```python
from build123d import *

# Parameters (mm, degrees)
SKETCH1_R           = 1.524
SKETCH1_R_2         = 2.4892
SKETCH1_R_3         = 11.522750336
SKETCH1_R_4         = 3.302
BOSS_EXTRUDE1_DEPTH = 6.35
CHAMFER1_SIZE       = 1.905
SKETCH2_R           = 1.1303
CUT_EXTRUDE1_DEPTH  = 12.7


with BuildPart() as part:
    # Sketch1 → Boss-Extrude1 (new body)
    with BuildSketch(Plane(origin=(0, 0, 0), x_dir=(1, 0, 0), z_dir=(0, 1, 0))):
        with BuildLine():
            Line((-48.989983611, 25.571283439), (-67.720507172, 29.04547214))
            Line((-67.720507172, 29.04547214), (-68.878570072, 22.801964286))
            Line((-68.878570072, 22.801964286), (-87.609093633, 26.276152988))
            Line((-87.609093633, 26.276152988), (-86.451030733, 32.519660841))
            Line((-86.451030733, 32.519660841), (-105.181554294, 35.993849543))
            Line((-105.181554294, 35.993849543), (-123.386535507, 39.370559213))
            Line((-123.386535507, 39.370559213), (-143.61245558, 43.122118146))
            Line((-143.61245558, 43.122118146), (-173.397808446, 32.126880331))
            Line((-173.397808446, 32.126880331), (-164.230158466, -34.209448348))
            Line((-164.230158466, -34.209448348), (-143.692879271, -77.813892282))
            Line((-143.692879271, -77.813892282), (-76.563330949, -77.813892282))
            Line((-76.563330949, -77.813892282), (-49.204879271, -77.813892282))
            Line((-49.204879271, -77.813892282), (-49.204879271, -37.681892282))
            Line((-49.204879271, -37.681892282), (45.277962712, -37.681892282))
            Line((45.277962712, -37.681892282), (64.72671994, -37.681892282))
            ThreePointArc((64.72671994, -37.681892282), (47.456106683, -24.721818432), (40.256527969, -4.364911427))
            ThreePointArc((40.256527969, -4.364911427), (40.224315343, -2.464216219), (40.304028245, -0.564920092))
            ThreePointArc((40.304028245, -0.564920092), (40.358687129, 0.79375425), (40.328560009, 2.153193811))
            ThreePointArc((40.328560009, 2.153193811), (38.274981353, 12.886225143), (33.41911498, 22.675796566))
            ThreePointArc((33.41911498, 22.675796566), (30.929713329, 27.951337515), (30.171477502, 33.73524029))
            ThreePointArc((30.171477502, 33.73524029), (27.651370411, 37.853265988), (22.862043617, 37.243820127))
            ThreePointArc((22.862043617, 37.243820127), (20.166682607, 36.055874133), (17.256896531, 36.513401897))
            ThreePointArc((17.256896531, 36.513401897), (8.843040964, 39.405959226), (0, 40.386))
            ThreePointArc((0, 40.386), (-9.489488111, 40.375548652), (-18.94466273, 39.569219451))
            ThreePointArc((-18.94466273, 39.569219451), (-22.43398811, 39.812343861), (-25.563809609, 41.373983535))
            ThreePointArc((-25.563809609, 41.373983535), (-32.045487778, 43.349075748), (-38.20024979, 40.514989348))
            ThreePointArc((-38.20024979, 40.514989348), (-40.550934903, 36.930082806), (-41.360215512, 32.720291801))
            ThreePointArc((-41.360215512, 32.720291801), (-43.17208429, 27.008072674), (-48.989983611, 25.571283439))
        make_face()
        with Locations(Location((-131.808500509, 37.703534036, 0), (0, 0, 270))):
            Circle(SKETCH1_R, mode=Mode.SUBTRACT)
        with Locations(Location((-31.399492492, 33.846007028, 0), (0, 0, 270))):
            Circle(SKETCH1_R, mode=Mode.SUBTRACT)
        with Locations(Location((-23.788932991, -8.902059713, 0), (0, 0, 270))):
            Circle(SKETCH1_R_2, mode=Mode.SUBTRACT)
        with Locations(Location((8.902059713, -23.788932991, 0), (0, 0, 270))):
            Circle(SKETCH1_R_2, mode=Mode.SUBTRACT)
        with Locations(Location((-8.902059713, 23.788932991, 0), (0, 0, 270))):
            Circle(SKETCH1_R_2, mode=Mode.SUBTRACT)
        with Locations(Location((23.788932991, 8.902059713, 0), (0, 0, 270))):
            Circle(SKETCH1_R_2, mode=Mode.SUBTRACT)
        with Locations(Location((0, 0, 0), (0, 0, 270))):
            Circle(SKETCH1_R_3, mode=Mode.SUBTRACT)
        with Locations(Location((-74.604879271, -57.747892282, 0), (0, 0, 270))):
            Circle(SKETCH1_R_4, mode=Mode.SUBTRACT)
        with Locations(Location((-40.020695033, -13.367428306, 0), (0, 0, 270))):
            Circle(SKETCH1_R, mode=Mode.SUBTRACT)
        with Locations(Location((25.727857837, 33.846007028, 0), (0, 0, 270))):
            Circle(SKETCH1_R, mode=Mode.SUBTRACT)
        with BuildLine():
            Line((-142.716614997, 32.622661546), (-162.215024972, 25.424839998))
            Line((-162.215024972, 25.424839998), (-156.726187504, -14.291916991))
            ThreePointArc((-156.726187504, -14.291916991), (-128.01028366, 5.891204618), (-94.602827713, 16.657049623))
            ThreePointArc((-94.602827713, 16.657049623), (-91.648290045, 20.089389422), (-94.519859105, 23.59143746))
            Line((-94.519859105, 23.59143746), (-142.716614997, 32.622661546))
        make_face(mode=Mode.SUBTRACT)
        with BuildLine():
            Line((-114.508797405, -72.415483536), (-119.588797405, -72.415483536))
            ThreePointArc((-119.588797405, -72.415483536), (-124.351297405, -67.652983536), (-119.588797405, -62.890483536))
            Line((-119.588797405, -62.890483536), (-114.508797405, -62.890483536))
            ThreePointArc((-114.508797405, -62.890483536), (-109.746297405, -67.652983536), (-114.508797405, -72.415483536))
        make_face(mode=Mode.SUBTRACT)
        with BuildLine():
            ThreePointArc((-147.948535824, -23.470306336), (-122.347176599, -5.47625853), (-92.563113904, 4.121916294))
            ThreePointArc((-92.563113904, 4.121916294), (-89.845720269, 1.990682905), (-91.74722838, -0.892137038))
            ThreePointArc((-91.74722838, -0.892137038), (-120.081933775, -10.023243789), (-144.437475152, -27.141662075))
            ThreePointArc((-144.437475152, -27.141662075), (-147.689154448, -26.736809805), (-147.948535824, -23.470306336))
        make_face(mode=Mode.SUBTRACT)
    extrude(amount=BOSS_EXTRUDE1_DEPTH)

    # Chamfer1
    # the kernel refuses this chamfer: 1.905 mm, written as the material it takes off along each edge
    with BuildSketch(Plane(origin=(-131.808500509, 0, -37.703534036), x_dir=(0, 0, 1), z_dir=(-1, 0, 0))) as chamfer1_piece_1:
        Polygon((1.524, CHAMFER1_SIZE), (1.524 + CHAMFER1_SIZE, 0), (1.524, 0), align=None)
    revolve(axis=Axis((-131.808500509, 0, -37.703534036), (0, 1, 0)), mode=Mode.SUBTRACT)
    with BuildSketch(Plane(origin=(-40.020695033, 0, 13.367428306), x_dir=(0, 0, 1), z_dir=(-1, 0, 0))) as chamfer1_piece_2:
        Polygon((1.524, CHAMFER1_SIZE), (1.524 + CHAMFER1_SIZE, 0), (1.524, 0), align=None)
    revolve(axis=Axis((-40.020695033, 0, 13.367428306), (0, 1, 0)), mode=Mode.SUBTRACT)
    with BuildSketch(Plane(origin=(25.727857837, 0, -33.846007028), x_dir=(0, 0, 1), z_dir=(-1, 0, 0))) as chamfer1_piece_3:
        Polygon((1.524, CHAMFER1_SIZE), (1.524 + CHAMFER1_SIZE, 0), (1.524, 0), align=None)
    revolve(axis=Axis((25.727857837, 0, -33.846007028), (0, 1, 0)), mode=Mode.SUBTRACT)
    with BuildSketch(Plane(origin=(-31.399492492, 0, -33.846007028), x_dir=(0, 0, 1), z_dir=(-1, 0, 0))) as chamfer1_piece_4:
        Polygon((1.524, CHAMFER1_SIZE), (1.524 + CHAMFER1_SIZE, 0), (1.524, 0), align=None)
    revolve(axis=Axis((-31.399492492, 0, -33.846007028), (0, 1, 0)), mode=Mode.SUBTRACT)

    # Sketch2 → Cut-Extrude1 (cut)
    with BuildSketch(Plane(origin=(1.797830768, 0, -9.692712298), x_dir=(-0.9832295832535866, 0, -0.18237211029918626), z_dir=(0.18237211029918626, 0, -0.9832295832535866))):
        with Locations((81.406890093, 3.175)):
            Circle(SKETCH2_R)
    extrude(amount=-CUT_EXTRUDE1_DEPTH, mode=Mode.SUBTRACT)


solid = part.part
```
The listing builds one solid part. Answer for the finished solid, in the listing's coordinates (mm). A direction names the side the tool comes from. Give positions to 0.01 mm unless a question says otherwise; leave off trailing zeros. Order: outer loops, then holes, each group sorted by start corner. A loop starts at its lowest first (then second) coordinate and runs counter-clockwise, first axis right, second up. Notation, with made-up numbers: M 84.25,21 L 142.25,21 A30 cw 142.25,53 Z; hole C 53,20.5 d6. An arc over 180 degrees is marked long. Put each result on its own line as item: value. Start each with the question number.
Item 1: Find the intervals of material crossed by line 1 along X through (y, z) = (1.25, -7); line 2 along Z through (x, y) = (-126, 3.75); line 3 along Z through (x, y) = (1, 5.75), in increasing order.
Item 2: The part is cut by section A-A, the plane x = -102. Determine the outline of the cut face in (y, z), and give its area (3 significant figures).
Item 3: For a pull along Y with two mould halves and no side action, classify faces 1 (the face through (-80.446, 3.515, -18.58)), 2 (the face through (-49.205, 3, 58)), 3 (the face through (-56, 0, 16)) as +Y half, -Y half, draft (parallel to the pull), parting line (faces both ways), or undercut.
Item 4: Flat-ended cylindrical pins translate along their axes: P1, Ø4, axis at x = 25.73, z = -33.85, coming from the -Y side; P2, Ø1.9, axis at x = 19.5, y = 3, coming from the +Z side; P3, Ø1.5, axis at x = -140, y = 3, coming from the -Z side. Find the tip coordinate at first contact, or state that the pin passes through.
Item 5: Which of the six approach directions +Z, -Z, +X, -X, +Y, -Y give full straight-line access (tool end or side, diameter ignored) to faces 4 (the face through (-158.3, 3.1, -37.7)), 5 (the face through (-87.04, 3.13, -29.35))?
Answer key:
1. line 1: x = -169.93 to -159.67, -125.72 to -9.15, 9.15 to 22.18, 25.39 to 39.77
1. line 2: z = -39.86 to -29.49, -6.87 to 7.39, 13.23 to 77.81
1. line 3: z = -40.37 to -11.48, 11.48 to 37.68
2. outline: M 0,-35.4 L 6.35,-35.4 L 6.35,-24.99 L 0,-24.99 Z; M 0,-15.21 L 6.35,-15.21 L 6.35,-2.14 L 0,-2.14 Z; M 0,3.12 L 6.35,3.12 L 6.35,77.81 L 0,77.81 Z
2. area: 623 mm²
3. face 1: undercut
3. face 2: draft
3. face 3: -Y half
4. P1: stops at y = 1.42
4. P2: stops at z = 37.68
4. P3: stops at z = -42.59
5. face 4: -Z, -X, +Y, -Y
5. face 5: +Y, -Y
